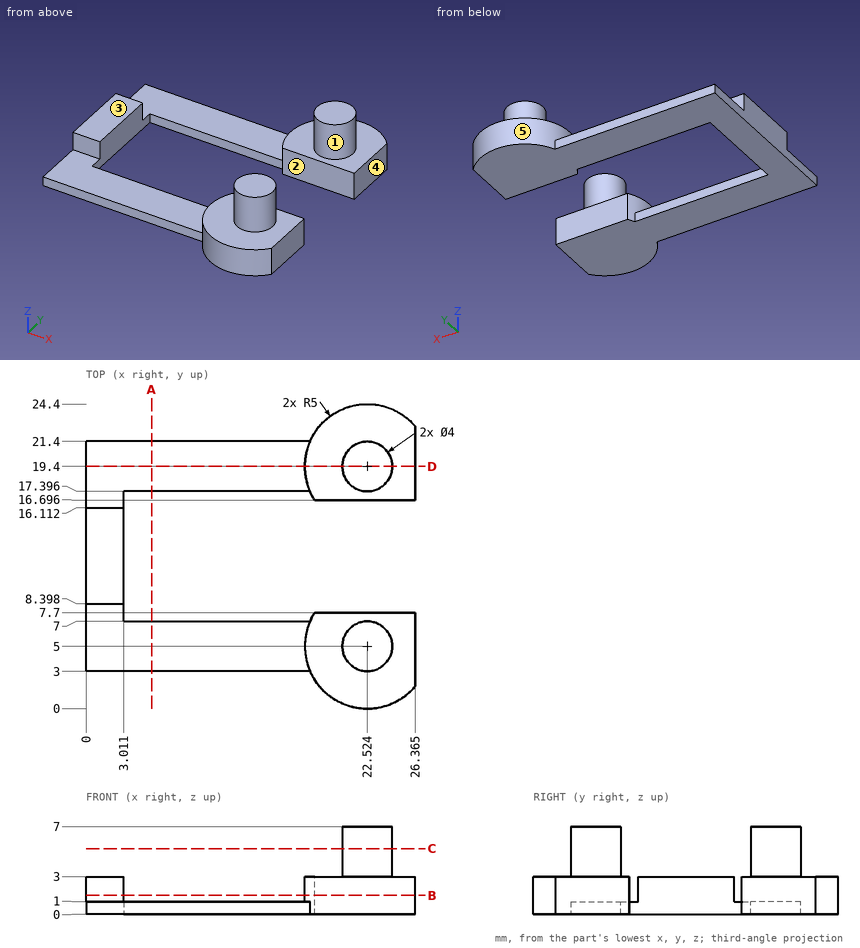
Could you check a few things on this drawing? It's one solid part, dimensions in mm from its lowest x, y, z. A direction names the side the tool comes from. Round coordinates to 2 decimals unless told otherwise and drop trailing zeros. Write each loop counter-clockwise with the first axis right and the second up, starting at its lowest first coordinate (ties: lowest second). Pieces come first, ordered by that corner, then holes. Notation, with made-up numbers: (-10.5, 11.5) -> (6.5, 11.5) arc R17 ccw to (6.5, 17.5) -> close; hole circle Ø1 at (-25, 46). An arc over 180 degrees is marked (long way). One line per question, with ' | ' between items. Start each with the question number.
1) Suppose I cut it at A-A on x = 5.25. Write out the boundary of the cut face in (y, z).
2) Suppose I cut it at C-C on z = 5.25. Write out the boundary of the cut face in (x, y).
3) On a 3-axis mill with a long thin cutter (end or side, diameter ignored), from which of +Z, -Z, +X, -X, +Y, -Y can I reach the whole of each face in a straight line? I mean the marked faces 1, 2 and 3. Say none if no direction works.
4) Suppose I cut it at D-D on y = 19.4. Write out the boundary of the cut face in (x, z) (1 decimal).
5) If we mould it in two halves opening along Y, with no side actions, what happens to the marked faces 4 and 5? For each: released by +Y, released by -Y, zero draft, split by the parting line, or undercut.
6) I need wall thicknesses on line 1 (Y direction, x = 22.5, z = 0.5); line 2 (Y direction, x = 11.25, z = 0.5); line 3 (Z direction, x = 6.5, y = 3.75). Which ranges of each line are inside material? Lowest first, please. Write a range as [from, to].
7) Suppose I cut it at B-B on z = 1.5. Write out the boundary of the cut face in (x, y) (1 decimal), then the cut area to 3 significant figures.
8) I'm going to push flat-ended pins straight in: P1, Ø1.6, axis at x = 2, z = 2, coming from the -Y side; P2, Ø0.5, axis at x = 10, z = 0.5, coming from the +Y side; P3, Ø2, axis at y = 2.5, z = 6, coming from the +X side (1 decimal). Where does each tip first touch, or does it pass through?
Return value:
1) outline: (3, 0) -> (7, 0) -> (7, 1) -> (3, 1) -> close; (17.4, 0) -> (21.4, 0) -> (21.4, 1) -> (17.4, 1) -> close
2) outline: circle Ø4 at (22.52, 5); circle Ø4 at (22.52, 19.4)
3) face 1: +Z | face 2: +Z, -Z, +X | face 3: +Z, +X, -X, +Y, -Y
4) outline: (0, 0) -> (26.4, 0) -> (26.4, 3) -> (24.5, 3) -> (24.5, 7) -> (20.5, 7) -> (20.5, 3) -> (17.5, 3) -> (17.5, 1) -> (0, 1) -> close
5) face 4: zero draft | face 5: undercut
6) line 1: y = [0, 7.7], [16.7, 24.4] | line 2: y = [3, 7], [17.4, 21.4] | line 3: z = [0, 1]
7) outline: (0, 8.4) -> (3, 8.4) -> (3, 16.1) -> (0, 16.1) -> close; (18.3, 7.7) arc R5 ccw to (26.4, 1.8) -> (26.4, 7.7) -> close; (18.3, 16.7) -> (26.4, 16.7) -> (26.4, 22.6) arc R5 ccw to start | area: 143 mm2
8) P1: stops at y = 8.4 | P2: stops at y = 21.4 | P3: stops at x = 23.8
